from build123d import *

# Parameters (mm, degrees)
CROQUIS1_W              = 120
CROQUIS1_H              = 80
SALIENTE_EXTRUIR1_DEPTH = 10
REDONDEO1_R             = 20
CROQUIS2_R              = 30
SALIENTE_EXTRUIR3_DEPTH = 120
CROQUIS6_R              = 15
SALIENTE_EXTRUIR4_DEPTH = 59
CROQUIS7_R              = 7.5
CORTAR_EXTRUIR1_DEPTH   = 64
CROQUIS8_R              = 15
CORTAR_EXTRUIR2_DEPTH   = 150
CROQUIS9_R              = 7.5
CORTAR_EXTRUIR3_DEPTH   = 83
CROQUIS10_R             = 15
SALIENTE_EXTRUIR5_DEPTH = 61
CROQUIS11_R             = 7.5
CORTAR_EXTRUIR4_DEPTH   = 78
CROQUIS12_R             = 15
CORTAR_EXTRUIR5_DEPTH   = 134


with BuildPart() as part:
    # Croquis1 → Saliente-Extruir1 (new body)
    with BuildSketch(Plane(origin=(0, 0, 0), x_dir=(1, 0, 0), z_dir=(0, 1, 0))):
        Rectangle(CROQUIS1_W, CROQUIS1_H)
    extrude(amount=SALIENTE_EXTRUIR1_DEPTH)

    # Redondeo1
    redondeo1_edges = [part.edges().sort_by_distance(p)[0] for p in [
        (60, 5, 40),
        (-60, 5, 40),
        (-60, 5, -40),
        (60, 5, -40),
    ]]
    fillet(redondeo1_edges, radius=REDONDEO1_R)

    # Croquis2 → Saliente-Extruir3 (add)
    with BuildSketch(Plane(origin=(0, 0, 0), x_dir=(1, 0, 0), z_dir=(0, 1, 0))):
        with Locations(Location((0, 0, 0), (0, 0, 90))):
            Circle(CROQUIS2_R)
    extrude(amount=SALIENTE_EXTRUIR3_DEPTH)

    # Croquis6 → Saliente-Extruir4 (add)
    with BuildSketch(Plane(origin=(79.319805153, 79.319805153, 0), x_dir=(0, 0, -1), z_dir=(0.7071067811865487, 0.7071067811865464, 0))):
        with Locations(Location((0, 24.748737342, 0), (0, 0, 90))):
            Circle(CROQUIS6_R)
    extrude(amount=-SALIENTE_EXTRUIR4_DEPTH)

    # Croquis7 → Cortar-Extruir1 (cut)
    with BuildSketch(Plane(origin=(79.319805153, 79.319805153, 0), x_dir=(0, 0, -1), z_dir=(0.7071067811865487, 0.7071067811865464, 0))):
        with Locations(Location((0, 24.748737342, 0), (0, 0, 90))):
            Circle(CROQUIS7_R)
    extrude(amount=-CORTAR_EXTRUIR1_DEPTH, mode=Mode.SUBTRACT)

    # Croquis8 → Cortar-Extruir2 (cut)
    with BuildSketch(Plane(origin=(0, 120, 0), x_dir=(1, 0, 0), z_dir=(0, 1, 0))):
        with Locations(Location((0, 0, 0), (0, 0, 270))):
            Circle(CROQUIS8_R)
    extrude(amount=-CORTAR_EXTRUIR2_DEPTH, mode=Mode.SUBTRACT)

    # Croquis9 → Cortar-Extruir3 (cut)
    with BuildSketch(Plane(origin=(79.319805153, 79.319805153, 0), x_dir=(0, 0, -1), z_dir=(0.7071067811865487, 0.7071067811865464, 0))):
        with Locations(Location((0, 24.748737342, 0), (0, 0, 90))):
            Circle(CROQUIS9_R)
    extrude(amount=-CORTAR_EXTRUIR3_DEPTH, mode=Mode.SUBTRACT)

    # Croquis10 → Saliente-Extruir5 (add)
    with BuildSketch(Plane(origin=(-79.319805153, 79.319805153, 0), x_dir=(0.7071067811865477, 0.7071067811865475, 0), z_dir=(-0.7071067811865475, 0.7071067811865477, 0))):
        with Locations(Location((24.748737342, 0, 0), (0, 0, 180))):
            Circle(CROQUIS10_R)
    extrude(amount=-SALIENTE_EXTRUIR5_DEPTH)

    # Croquis11 → Cortar-Extruir4 (cut)
    with BuildSketch(Plane(origin=(-79.319805153, 79.319805153, 0), x_dir=(0.7071067811865477, 0.7071067811865475, 0), z_dir=(-0.7071067811865475, 0.7071067811865477, 0))):
        with Locations(Location((24.748737342, 0, 0), (0, 0, 180))):
            Circle(CROQUIS11_R)
    extrude(amount=-CORTAR_EXTRUIR4_DEPTH, mode=Mode.SUBTRACT)

    # Croquis12 → Cortar-Extruir5 (cut)
    with BuildSketch(Plane(origin=(0, 120, 0), x_dir=(1, 0, 0), z_dir=(0, 1, 0))):
        with Locations(Location((0, 0, 0), (0, 0, 270))):
            Circle(CROQUIS12_R)
    extrude(amount=-CORTAR_EXTRUIR5_DEPTH, mode=Mode.SUBTRACT)


solid = part.part
Can you work these out from the model? Positions are in its coordinate system, mm. A direction names the side the tool comes from. Coordinates: 2 decimals unless noted, no trailing zeros. Loops run counter-clockwise (first coordinate to the right, second up) from the corner with the lowest first, then second, coordinate; pieces in that order, holes last. Notation, with made-up numbers: (-36.75, 28) - (20.25, 28) arc R30 ccw to (20.25, 60) - close; hole circle Ø9 at (27.5, 57.25). An arc over 180 degrees is marked (long way). Put each result on its own line as item: value. Start each with the question number.
Item 1: Suppose I cut it at A-A (x = 5). Please give me the cut outline in (y, z), and give its area (3 significant figures).
Item 2: Suppose I cut it at D-D (z = 32). Please give me the cut outline in (x, y).
Item 3: If we mould it in two halves opening along Y, with no side actions, what happens to faces 5 (the face through (-56.96, 101.68, 3.54)), 6 (the face through (-14, 10, -27)), 7 (the face through (14.872, 60.84, -1.953))? For each: +Y half, -Y half, draft (parallel to the pull), parting line (faces both ways), or undercut.
Item 4: For pin 1 (8 mm diameter, centred on x = 15.5, y = 91.5, fed in from +Z); pin 2 (10 mm diameter, centred on x = -35, z = 0.5, fed in from -Y); pin 3 (10 mm diameter, centred on x = 57.5, y = 66, fed in from +Z); pin 4 (5 mm diameter, centred on y = 6.5, z = -2, fed in from +X), each with a flat end and sliding along its axis, tell me the tip position at first contact or that it passes through.
Item 5: If I drill on line 1 along X through (y, z) = (37, 0); line 2 along X through (y, z) = (78, -3.5); line 3 along X through (y, z) = (93, 0), over which ranges is the centre line in solid material (lowest first)?
Item 6: Suppose I cut it at C-C (y = 25.5). Please give me the cut outline in (x, z).
Item 7: Suppose I cut it at B-B (z = 0). State how many separate pieces and enclosed holes the cut face has, and give its area (3 significant figures).
Item 8: Which directions (+Z, -Z, +X, -X, +Y, -Y) give clear straight access to the entire face, cutting with the end or side of a thin tool? Please do faces 1 (the face through (-25.296, 64.23, -16.128)), 2 (the face through (53.986, 5.07, 34.297)), 3 (the face through (60, 5, 0)), 4 (the face through (-60, 5, 0)).
Here are the results:
1. outline: (0, -40) - (10, -40) - (10, -29.58) - (120, -29.58) - (120, -14.14) - (0, -14.14) - close; (0, 14.14) - (120, 14.14) - (120, 29.58) - (10, 29.58) - (10, 40) - (0, 40) - close
1. area: 3,910 mm²
2. outline: (-56, 0) - (56, 0) - (56, 10) - (-56, 10) - close
3. face 5: +Y half
3. face 6: undercut
3. face 7: draft
4. pin 1: z = 27.71
4. pin 2: y = 0
4. pin 3: z = 6.02
4. pin 4: x = 60
5. line 1: -30 to -15, 15 to 30
5. line 2: -63.63 to -52.38, -33.62 to -14.59, 14.59 to 33.62, 52.38 to 63.63
5. line 3: -47.39 to -36.79, -30 to -15, 15 to 30, 36.79 to 47.39
6. outline: circle Ø60 at (0, 0); hole circle Ø30 at (0, 0)
7. separate pieces: 4
7. enclosed holes: 0
7. area: 4,910 mm²
8. face 1: none
8. face 2: +Z, +X, +Y, -Y
8. face 3: +Z, -Z, +X, -Y
8. face 4: +Z, -Z, -X, -Y
